Geometry: see drawing. Coordinates: mm, zero at the bounding-box minimum. A direction names the side the tool comes from. Coordinates: 2 decimals unless noted, no trailing zeros. Write each loop counter-clockwise with the first axis right and the second up, starting at its lowest first coordinate (ties: lowest second). Pieces come first, ordered by that corner, then holes. Notation, with made-up numbers: (80, 75.5) -> (116, 75.5) arc R11 ccw to (116, 90.5) -> close; hole circle Ø4 at (22.5, 86.25). An arc over 180 degrees is marked (long way). Use one line per item in the form item = value. Start each with the question number.
(1) Cut plane D-D on y = 11.5. Return the cut outline in (x, z).
(2) Cut plane C-C on y = 1.75. Return the cut outline in (x, z), plus the area to 3 significant figures.
(3) Cut plane B-B on x = 4.25. Return the cut outline in (y, z).
(4) Set-up query: the marked faces 4, 5 and 6. Return all of +Z, -Z, +X, -X, +Y, -Y with unobstructed straight access to the full face (end or side cutting, diameter ignored); none if empty.
(5) First-contact query: pin 1 (4 mm diameter, centred on y = 7.5, z = 4, fed in from -X); pin 2 (2 mm diameter, centred on y = 9.5, z = 2, fed in from +X); pin 3 (1 mm diameter, centred on y = 11, z = 2, fed in from +X). Flat tips, straight axial feed; report the tip coordinate or a pass-through.
(6) Pull-direction query (Z, two-part tool) for the marked faces 1, 2 and 3; classes: released by +Z, released by -Z, zero draft, split by the parting line, or undercut.
(7) Ray query, line 1 along Z through (x, y) = (8, 13.75); line 2 along Y through (x, z) = (2, 2); line 3 along Z through (x, y) = (4.25, 14.75). Return the intervals inside material, ascending.
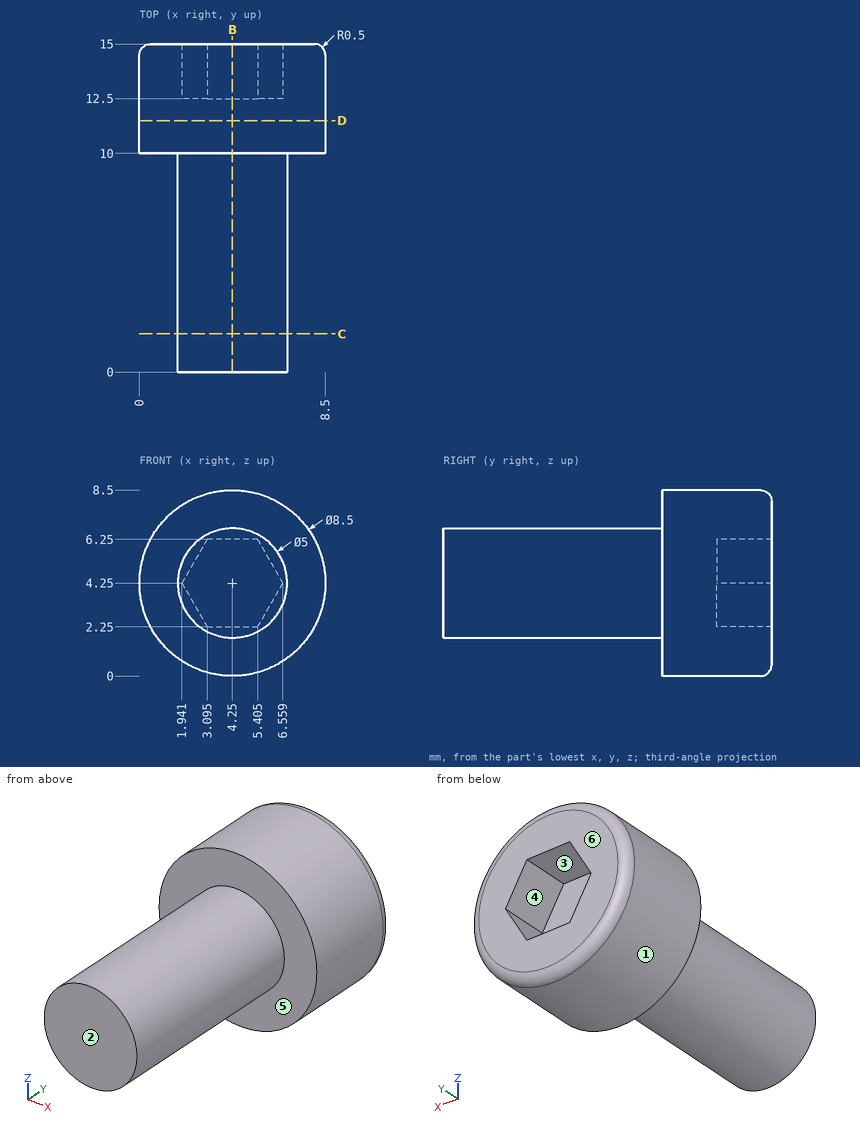
Values:
q1.outline = circle Ø8.5 at (4.25, 4.25)
q2.outline = circle Ø5 at (4.25, 4.25)
q2.area = 19.6 mm2
q3.outline = (0, 1.75) -> (10, 1.75) -> (10, 0) -> (14.5, 0) arc R0.5 ccw to (15, 0.5) -> (15, 2.25) -> (12.5, 2.25) -> (12.5, 6.25) -> (15, 6.25) -> (15, 8) arc R0.5 ccw to (14.5, 8.5) -> (10, 8.5) -> (10, 6.75) -> (0, 6.75) -> close
q4.face_4 = +Y
q4.face_5 = -Y
q4.face_6 = +Z, -Z, +X, -X, +Y
q5.pin_1 = 1.75
q5.pin_2 = 8.27
q5.pin_3 = 8.12
q6.face_1 = split by the parting line
q6.face_2 = zero draft
q6.face_3 = undercut
q7.line_1 = 2.25 to 6.25
q7.line_2 = 10 to 15
q7.line_3 = 0.07 to 2.25, 6.25 to 8.43
